Part model, mm, in its own coordinate system. Face numbers are marked on the shaded views. Give positions to 0.01 mm unless a question says otherwise; leave off trailing zeros. Order: outer loops, then holes, each group sorted by start corner. A loop starts at its lowest first (then second) coordinate and runs counter-clockwise, first axis right, second up. Notation, with made-up numbers: (57.5, 42) - (84.5, 42) arc R29 ccw to (84.5, 62) - close; hole circle Ø4 at (53, 39.25). An arc over 180 degrees is marked (long way). Use a Markdown table: item, result. Add a question column.
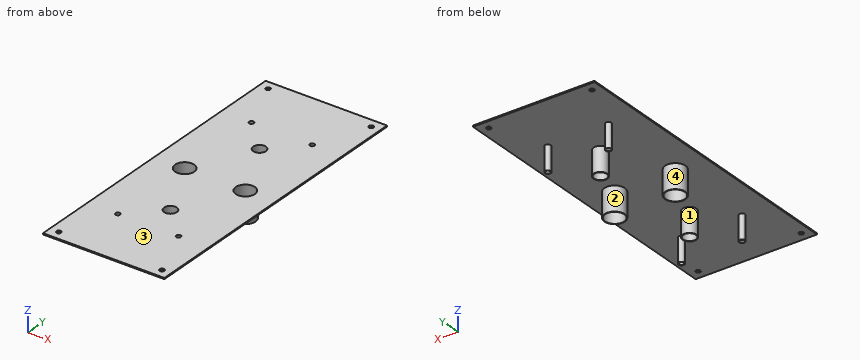
from build123d import *

# Parameters (mm, degrees)
F0_W     = 1000
F0_H     = 2500
F0_R     = 19.15
F0_R_2   = 52.15
F0_R_3   = 79.15
F1_DEPTH = 10
F2_R     = 24
F2_R_2   = 19.15
F2_R_3   = 57.15
F2_R_4   = 52.15
F2_R_5   = 84.15
F2_R_6   = 79.15
F3_DEPTH = 200


with BuildPart() as f1:
    # F0 (on Top) → F1 (new body)
    with BuildSketch(Plane.XY):
        Rectangle(F0_W, F0_H)
        with Locations((-425, -1175)):
            Circle(F0_R, mode=Mode.SUBTRACT)
        with Locations((-250, -750)):
            Circle(F0_R, mode=Mode.SUBTRACT)
        with Locations((425, -1175)):
            Circle(F0_R, mode=Mode.SUBTRACT)
        with Locations((250, -750)):
            Circle(F0_R, mode=Mode.SUBTRACT)
        with Locations((0, -500)):
            Circle(F0_R_2, mode=Mode.SUBTRACT)
        with Locations((-250, 0)):
            Circle(F0_R_3, mode=Mode.SUBTRACT)
        with Locations((-425, 1175)):
            Circle(F0_R, mode=Mode.SUBTRACT)
        with Locations((-250, 750)):
            Circle(F0_R, mode=Mode.SUBTRACT)
        with Locations((0, 500)):
            Circle(F0_R_2, mode=Mode.SUBTRACT)
        with Locations((250, 0)):
            Circle(F0_R_3, mode=Mode.SUBTRACT)
        with Locations((250, 750)):
            Circle(F0_R, mode=Mode.SUBTRACT)
        with Locations((425, 1175)):
            Circle(F0_R, mode=Mode.SUBTRACT)
    extrude(amount=F1_DEPTH)

    # F2 (on face) → F3 (join)
    with BuildSketch(Plane(origin=(0, 0, 0), x_dir=(1, 0, 0), z_dir=(0, 0, -1))):
        with Locations((250, 750)):
            Circle(F2_R)
        with Locations((250, 750)):
            Circle(F2_R_2, mode=Mode.SUBTRACT)
        with Locations((-250, 750)):
            Circle(F2_R)
        with Locations((-250, 750)):
            Circle(F2_R_2, mode=Mode.SUBTRACT)
        with Locations((0, 500)):
            Circle(F2_R_3)
        with Locations((0, 500)):
            Circle(F2_R_4, mode=Mode.SUBTRACT)
        with Locations((250, 0)):
            Circle(F2_R_5)
        with Locations((250, 0)):
            Circle(F2_R_6, mode=Mode.SUBTRACT)
        with Locations((0, -500)):
            Circle(F2_R_3)
        with Locations((0, -500)):
            Circle(F2_R_4, mode=Mode.SUBTRACT)
        with Locations((250, -750)):
            Circle(F2_R)
        with Locations((250, -750)):
            Circle(F2_R_2, mode=Mode.SUBTRACT)
        with Locations((-250, -750)):
            Circle(F2_R)
        with Locations((-250, -750)):
            Circle(F2_R_2, mode=Mode.SUBTRACT)
        with Locations((-250, 0)):
            Circle(F2_R_5)
        with Locations((-250, 0)):
            Circle(F2_R_6, mode=Mode.SUBTRACT)
    extrude(amount=F3_DEPTH)


solid = f1.part
1. Cut at C-C (x = 0). Write the cut outline in (y, z).
2. Cut at D-D (y = 0). Write the cut outline in (x, z), plus the area to 3 significant figures.
3. Pin check, flat tips, straight feed: P1, Ø3, axis at x = 189.5, y = -113.5, coming from the -Z side; P2, Ø3, axis at x = 264, z = -14, coming from the -Y side. Stop position of each tip, or through.
4. Cut at B-B (y = -500). Write the cut outline in (x, z).
5. Mould opens along X. For the marked faces 1, 2, 3 and 4 say: released by +X, released by -X, zero draft, split by the parting line, or undercut.
6. Cut at A-A (z = -24). State how many separate pieces and enclosed holes the cut face has, plus the area to 3 significant figures.
7. Drill centre lines: probe 1 along X at (y, z) = (1175, 2.5); probe 2 along Y at (x, z) = (0, -87); probe 3 along X at (y, z) = (-500, -55). Where is each one in solid material? Low to high. Write a range as [from, to].
Responses:
| question | item | result |
|---|---|---|
| 1 | outline | (-1250, 0) - (-557.15, 0) - (-557.15, -200) - (-552.15, -200) - (-552.15, 10) - (-1250, 10) - close; (-447.85, -200) - (-442.85, -200) - (-442.85, 0) - (442.85, 0) - (442.85, -200) - (447.85, -200) - (447.85, 10) - (-447.85, 10) - close; (552.15, -200) - (557.15, -200) - (557.15, 0) - (1250, 0) - (1250, 10) - (552.15, 10) - close |
| 2 | outline | (-500, 0) - (-334.15, 0) - (-334.15, -200) - (-329.15, -200) - (-329.15, 10) - (-500, 10) - close; (-170.85, -200) - (-165.85, -200) - (-165.85, 0) - (165.85, 0) - (165.85, -200) - (170.85, -200) - (170.85, 10) - (-170.85, 10) - close; (329.15, -200) - (334.15, -200) - (334.15, 0) - (500, 0) - (500, 10) - (329.15, 10) - close |
| 2 | area | 10,800 mm² |
| 3 | P1 | stops at z = 0 |
| 3 | P2 | stops at y = -770.49 |
| 4 | outline | (-500, 0) - (-57.15, 0) - (-57.15, -200) - (-52.15, -200) - (-52.15, 10) - (-500, 10) - close; (52.15, -200) - (57.15, -200) - (57.15, 0) - (500, 0) - (500, 10) - (52.15, 10) - close |
| 5 | face 1 | split by the parting line |
| 5 | face 2 | undercut |
| 5 | face 3 | zero draft |
| 5 | face 4 | undercut |
| 6 | separate pieces | 8 |
| 6 | enclosed holes | 8 |
| 6 | area | 11,200 mm² |
| 7 | probe 1 | x = [-500, -444.15], [-405.85, 405.85], [444.15, 500] |
| 7 | probe 2 | y = [-557.15, -552.15], [-447.85, -442.85], [442.85, 447.85], [552.15, 557.15] |
| 7 | probe 3 | x = [-57.15, -52.15], [52.15, 57.15] |
